```python
from build123d import *

# Parameters (mm, degrees)
SKETCH_4_R          = 1.6
CUT_EXTRUDE_1_DEPTH = 10
CHAMFER_1_SIZE      = 0.5


with BuildPart() as part:
    # 草图3 → 旋转1 (revolve)
    with BuildSketch(Plane(origin=(0, 0, 0), x_dir=(0, 0, -1), z_dir=(1, 0, 0)), mode=Mode.PRIVATE) as revolve_1_sk:
        Polygon((-7.5, 0), (0, 0), (0, -4), (-4.125, -4), (-11, -48), (-15, -48), align=None)
    revolve(revolve_1_sk.sketch.rotate(Axis((0, 28.450677981, 0), (0, 1, 0)), 180), axis=Axis((0, 28.450677981, 0), (0, 1, 0)))

    # 草图4 → 切除-拉伸1 (cut)
    with BuildSketch(Plane(origin=(0, 0, 0), x_dir=(1, 0, 0), z_dir=(0, 1, 0))):
        with Locations(Location((0, 0, 0), (0, 0, 270))):
            Circle(SKETCH_4_R)
    extrude(amount=-CUT_EXTRUDE_1_DEPTH, mode=Mode.SUBTRACT)

    # 倒角1
    chamfer_1_edges = [part.edges().sort_by_distance(p)[0] for p in [
        (0, -4, -1.6),
        (0, 0, -1.6),
    ]]
    chamfer(chamfer_1_edges, length=CHAMFER_1_SIZE)


solid = part.part
```
Verification items for the finished model (mm, model axes). Give positions to 0.01 mm unless a question says otherwise; leave off trailing zeros. Order: outer loops, then holes, each group sorted by start corner. A loop starts at its lowest first (then second) coordinate and runs counter-clockwise, first axis right, second up. Notation, with made-up numbers: (-13, 16.5) -> (-1, 16.5) arc R28 ccw to (-1, 35.5) -> close; hole circle Ø11 at (46, -27). An arc over 180 degrees is marked (long way). One line per item, written item: value.
(1) Draft check along Z on faces 1 (the face through (-11.1, -23.66, 1.46)), 2 (the face through (2, 0, -2)), 3 (the face through (2, -4, 2)). Enter one of: pulls with the +Z half, pulls with the -Z half, needs draft (parallel to the pull), parting line crosses it, or undercut.
Final values:
face 1: parting line crosses it
face 2: needs draft
face 3: undercut
(2) Sectioned sample at B-B on x = 0. Record the cut outline in (y, z) (3 decimals), then the cut area to 3 significant figures.
Final values:
outline: (-48, -15) -> (0, -7.5) -> (0, -2.1) -> (-0.5, -1.6) -> (-3.5, -1.6) -> (-4, -2.1) -> (-4, -4.125) -> (-48, -11) -> close; (-48, 11) -> (-4, 4.125) -> (-4, 2.1) -> (-3.5, 1.6) -> (-0.5, 1.6) -> (0, 2.1) -> (0, 7.5) -> (-48, 15) -> close
area: 401 mm^2
(3) Sectioned sample at A-A on z = 0. Record the cut outline in (x, y) (3 decimals).
Final values:
outline: (-15, -48) -> (-11, -48) -> (-4.125, -4) -> (-2.1, -4) -> (-1.6, -3.5) -> (-1.6, -0.5) -> (-2.1, 0) -> (-7.5, 0) -> close; (1.6, -3.5) -> (2.1, -4) -> (4.125, -4) -> (11, -48) -> (15, -48) -> (7.5, 0) -> (2.1, 0) -> (1.6, -0.5) -> close
(4) Sectioned sample at C-C on y = -8. Record the cut outline in (x, z), then the cut area to 3 significant figures.
Final values:
outline: circle Ø17.5 at (0, 0); hole circle Ø9.5 at (0, 0)
area: 170 mm^2
(5) Sectioned sample at D-D on y = -36. Record the cut outline in (x, z) (3 decimals).
Final values:
outline: circle Ø26.25 at (0, 0); hole circle Ø18.25 at (0, 0)
(6) Scan lines: line 1 along X through (y, z) = (-29, 6.25); line 2 along X through (y, z) = (-18.5, -1.25); line 3 along Z through (x, y) = (5, -19). Record each from-to range of solid material in increasing order. Write a range as [from, to].
Final values:
line 1: [-10.28, -5.04], [5.04, 10.28]
line 2: [-10.32, -6.27], [6.27, 10.32]
line 3: [-9.2, -4.1], [4.1, 9.2]
(7) Gauge pin test, flat ends, axial feed: pin 1 (5 mm diameter, centred on y = -33.5, z = -4, fed in from -X); pin 2 (8 mm diameter, centred on y = -13, z = 0, fed in from +X); pin 3 (4 mm diameter, centred on x = -1, z = -0.5, fed in from -Y); pin 4 (3 mm diameter, centred on x = 0, z = 0, fed in from +Y). Record the tip position at first contact, or that the pin passes through.
Final values:
pin 1: x = -12.82
pin 2: x = 10.16
pin 3: y = -4
pin 4: through
